The listing builds one solid part. Answer for the finished solid, in the listing's coordinates (mm). A direction names the side the tool comes from. Give positions to 0.01 mm unless a question says otherwise; leave off trailing zeros. Order: outer loops, then holes, each group sorted by start corner. A loop starts at its lowest first (then second) coordinate and runs counter-clockwise, first axis right, second up. Notation, with made-up numbers: M -9.75,-23 L 37.25,-23 A26 ccw 37.25,0 Z; hole C 48.5,66.5 d1. An arc over 180 degrees is marked long. Answer as a JSON object with one key per item and string values. Group by question number.
```python
from build123d import *

# Parameters (mm, degrees)
BASPROSKE_W         = 6
BASPROSKE_H         = 12.375
TOOTHCUT_DEPTH      = 19.500844575
TEETHCUTS_COUNT     = 20
BORSKE_R            = 3
BORE_DEPTH          = 50.0000508
SKETCH1_R           = 3
BOSS_EXTRUDE1_DEPTH = 6
CUT_EXTRUDE1_DEPTH  = 6
SKETCH3_R           = 3
CUT_EXTRUDE2_DEPTH  = 6


with BuildPart() as part:
    # BasProSke → Base-Revolve (revolve)
    with BuildSketch(Plane(origin=(0, 0, 0), x_dir=(1, 0, 0), z_dir=(0, 1, 0)), mode=Mode.PRIVATE) as base_revolve_sk:
        with Locations((3, 6.1875)):
            Rectangle(BASPROSKE_W, BASPROSKE_H)
    revolve(base_revolve_sk.sketch.rotate(Axis((-10, 0, 0), (1, 0, 0)), 180), axis=Axis((-10, 0, 0), (1, 0, 0)))

    # TooCutSke → ToothCut (cut, through all)
    with BuildSketch(Plane(origin=(0, 0, 0), x_dir=(0, 0, -1), z_dir=(1, 0, 0))):
        with BuildLine():
            ThreePointArc((0.561279811, 9.826733564), (0, 9.84275), (-0.561279811, 9.826733564))
            ThreePointArc((-0.561279811, 9.826733564), (-0.925277854, 11.14210546), (-1.666860651, 12.287859689))
            ThreePointArc((-1.666860651, 12.287859689), (0, 12.4004), (1.666860651, 12.287859689))
            ThreePointArc((1.666860651, 12.287859689), (0.925277854, 11.14210546), (0.561279811, 9.826733564))
        make_face()
    toothcut = extrude(amount=TOOTHCUT_DEPTH, mode=Mode.SUBTRACT)

    # TeethCuts: ToothCut ×20 about axis
    teethcuts_axis = Axis((0, 0, 0), (1, 0, 0))
    for i in range(1, TEETHCUTS_COUNT):
        add(toothcut.rotate(teethcuts_axis, i * 360 / TEETHCUTS_COUNT), mode=Mode.SUBTRACT)

    # BorSke → Bore (cut, symmetric)
    with BuildSketch(Plane(origin=(0, 0, 0), x_dir=(0, 0, -1), z_dir=(1, 0, 0))):
        with Locations(Location((0, 0, 0), (0, 0, 180))):
            Circle(BORSKE_R)
    extrude(amount=BORE_DEPTH, both=True, mode=Mode.SUBTRACT)

    # Sketch1 → Boss-Extrude1 (add)
    with BuildSketch(Plane(origin=(6, 0, 0), x_dir=(0, 0, -1), z_dir=(1, 0, 0))):
        Circle(SKETCH1_R)
    extrude(amount=-BOSS_EXTRUDE1_DEPTH)

    # Sketch2 → Cut-Extrude1 (cut)
    with BuildSketch(Plane(origin=(6, 0, 0), x_dir=(0, 0, -1), z_dir=(1, 0, 0))):
        with BuildLine():
            ThreePointArc((1.8, 2.01246118), (0, 2.7), (-1.8, 2.01246118))
            Line((-1.8, 2.01246118), (-1.8, 0))
            Line((-1.8, 0), (1.8, 0))
            Line((1.8, 0), (1.8, 2.01246118))
        make_face()
        with BuildLine():
            Line((1.8, 0), (-1.8, 0))
            Line((-1.8, 0), (-1.8, -2.01246118))
            ThreePointArc((-1.8, -2.01246118), (0, -2.7), (1.8, -2.01246118))
            Line((1.8, -2.01246118), (1.8, 0))
        make_face()
    extrude(amount=-CUT_EXTRUDE1_DEPTH, mode=Mode.SUBTRACT)

    # Sketch3 → Cut-Extrude2 (cut)
    with BuildSketch(Plane(origin=(6, 0, 0), x_dir=(0, 0, -1), z_dir=(1, 0, 0))):
        Circle(SKETCH3_R)
    extrude(amount=-CUT_EXTRUDE2_DEPTH, mode=Mode.SUBTRACT)


solid = part.part
```
Item 1: Consider probe 1 along Z at (x, y) = (1.5, -8.25); probe 2 along Z at (x, y) = (1.5, 5.5); probe 3 along Y at (x, z) = (2.3, 9.75). Determine where each line is inside the solid, lowest interval first. Write a range as from..to.
Item 2: Section C-C (y = -6.75) is taken. Determine the outline of the cut face in (x, z), and give its area (3 significant figures).
Item 3: Section D-D (z = -4) is taken. Determine the outline of the cut face in (x, y).
Item 4: Flat-ended cylindrical pins translate along their axes: P1, Ø3, axis at x = 3, y = -8, coming from the +Z side; P2, Ø1.5, axis at x = 2, y = -8.5, coming from the -Z side. Find the tip coordinate at first contact, or state that the pin passes through.
Item 5: Section A-A (y = 0) is taken. Determine the outline of the cut face in (x, z), and give its area (3 significant figures).
Item 6: A tool of negligible diameter and unlimited length cuts with its end or side. For faces 1 (the cylindrical face through (2.96, -0.93, -11.15)), 2 (the cylindrical face through (2.96, -11.11, -0.91)), 3 (the cylindrical face through (2.96, -7.96, 5.79)), from which of +Z, -Z, +X, -X, +Y, -Y can it reach the whole face along a straight path? Write none if from no direction.
Item 7: Determine the mould class of faces 4 (the cylindrical face through (2.958, 4.3, -10.285)), 5 (the cylindrical face through (3, 0, 3)), 6 (the cylindrical face through (2.958, 4.326, 10.314)) for opening direction Z: released by +Z, released by -Z, zero draft, split by the parting line, or undercut.
Values found:
{
 "1": {"probe 1": "z = -8.88..-6.95, -5.37..5.37, 6.95..8.88", "probe 2": "z = -11.09..-8.63, -8.16..8.16, 8.63..11.09", "probe 3": "y = -5.84..-3.89, -2.54..2.54, 3.89..5.84"},
 "2": {"outline": "M 0,-8.1 L 6,-8.1 L 6,8.1 L 0,8.1 Z", "area": "97.2 mm^2"},
 "3": {"outline": "M 0,-9.91 L 6,-9.91 L 6,9.91 L 0,9.91 Z"},
 "4": {"P1": "stops at z = 8.95", "P2": "stops at z = -8.95"},
 "5": {"outline": "M 0,-9.84 L 6,-9.84 L 6,-3 L 0,-3 Z; M 0,3 L 6,3 L 6,9.84 L 0,9.84 Z", "area": "82.1 mm^2"},
 "6": {"face 1": "-Z, +X, -X", "face 2": "+X, -X, -Y", "face 3": "+X, -X"},
 "7": {"face 4": "released by -Z", "face 5": "undercut", "face 6": "released by +Z"}
}
